```python
from build123d import *

# Parameters (mm, degrees)
F0_W     = 50
F0_H     = 5
F2_DEPTH = 50


with BuildPart() as f1:
    # F0 (on Front) → F1 (revolve)
    with BuildSketch(Plane.XZ):
        Polygon((-29.5, 0), (-24.5, 0), (-24.5, 13), (-24.5, 30), (-29.5, 30), align=None)
        with BuildLine():
            Line((-24.5, 0), (-17.75, 0))
            ThreePointArc((-17.75, 0), (-22.711917, 5.676024), (-24.5, 13))
            Line((-24.5, 13), (-24.5, 0))
        make_face()
    revolve(axis=Axis((0, 0, -2.5), (0, 0, -1)))

    # F0 (on Front) → F2 (join, symmetric)
    with BuildSketch(Plane.XZ):
        Polygon((0, -5), (0, 0), (-17.75, 0), (-24.5, 0), (-29.5, 0), (-50, 0), (-50, -5), align=None)
        with Locations((25, -2.5)):
            Rectangle(F0_W, F0_H)
    extrude(amount=F2_DEPTH, both=True)


with BuildPart() as f3_1:
    # F3: copy of F1
    add(f1.part)


solid = f1.part
```
CAD build for the part. Positions are in the model's coordinates, mm. A direction names the side the tool comes from. Round coordinates to 2 decimals unless told otherwise and drop trailing zeros. Order: outer loops, then holes, each group sorted by start corner. A loop starts at its lowest first (then second) coordinate and runs counter-clockwise, first axis right, second up. Notation, with made-up numbers: (5, 75.5) -> (29, 75.5) arc R24 cw to (29, 93.5) -> close; hole circle Ø5 at (13.5, 79.25). An arc over 180 degrees is marked (long way). Write item = value, one per line.
(1) Drill centre lines: L1, parallel to Y at x = 0, z = 17.5; L2, parallel to Z at x = 2.5, y = 35.5; L3, parallel to X at y = 11, z = 1.5. Where is each one in solid material? Low to high.
Answers follow:
L1 = -29.5 to -24.5, 24.5 to 29.5
L2 = -5 to 0
L3 = -27.37 to -16.19, 16.19 to 27.37
(2) Cut at B-B (z = 21). Write the cut outline in (x, y), plus the area to 3 significant figures.
Answers follow:
outline = circle Ø59 at (0, 0); hole circle Ø49 at (0, 0)
area = 848 mm²
(3) 3-axis set-ups, long thin cutter, end or side, ignore diameter. For faces 1 (the cylindrical face through (-13.17, 20.66, 21.62)), 2 (the flat face through (-1, 50, -2)): which of +Z, -Z, +X, -X, +Y, -Y reach the whole face in a straight line?
Answers follow:
face_1 = +Z
face_2 = +Z, -Z, +X, -X, +Y
(4) Pull direction X, two halves, no side cores. Call faces 3 (the cylindrical face through (-28.14, 8.86, 14.79)), 4 (the flat face through (0, 0, 0)), 5 (the flat face through (-50, -1, -2)): +X half, -X half, draft (parallel to the pull), parting line (faces both ways), or undercut.
Answers follow:
face_3 = parting line
face_4 = undercut
face_5 = -X half
(5) Cut at A-A (y = 44). Write the cut outline in (x, z).
Answers follow:
outline = (-50, -5) -> (50, -5) -> (50, 0) -> (-50, 0) -> close
(6) Flat gauge pins, fed straight in: P1, Ø4, axis at x = 6, z = 14, coming from the +Y side; P2, Ø4, axis at y = -32.5, z = 23.5, coming from the +X side; P3, Ø6, axis at y = -19.5, z = 9, coming from the +X side. Where does each tip first touch, or does it go through?
Answers follow:
P1 = 29.23
P2 = through
P3 = 24.45
